CAD build for the part. Positions are in the model's coordinates, mm. A direction names the side the tool comes from. Give positions to 0.01 mm unless a question says otherwise; leave off trailing zeros. Order: outer loops, then holes, each group sorted by start corner. A loop starts at its lowest first (then second) coordinate and runs counter-clockwise, first axis right, second up. Notation, with made-up numbers: M 60,40.5 L 108,40.5 A27 cw 108,72.5 Z; hole C 73.5,-19.75 d2. An arc over 180 degrees is marked long. Put each result on its own line as item: value. Start each with the question number.
1) Cut at C-C (y = -19). Write the cut outline in (x, z), and give its area (3 significant figures).
2) Drill centre lines: line 1 (Z direction, x = 23, y = 12); line 2 (Y direction, x = 0, z = 4.5); line 3 (Y direction, x = -17.5, z = 1.25). Where is each one in solid material? Low to high. Write a range as [from, to].
3) Two-plate mould, pull along X, no slides. Class faces 1 (the face through (0, 0, 0)), 2 (the face through (-8.75, 28, 3)), 3 (the face through (0, 0, -2)): released by +X, released by -X, zero draft, split by the parting line, or undercut.
4) Cut at A-A (x = 0). Write the cut outline in (y, z), and give its area (3 significant figures).
5) Tool access for faces 4 (the face through (9, -27.5, 10)), 5 (the face through (8.75, 28, 3)): list every direction of +Z, -Z, +X, -X, +Y, -Y with a clear straight run to the whole face (end or side of a thin tool).
6) Cut at D-D (x = 20). Write the cut outline in (y, z), and give its area (3 significant figures).
7) Cut at B-B (z = 9.25). Write the cut outline in (x, y).
8) Pin check, flat tips, straight feed: pin 1 (1.6 mm diameter, centred on x = -3, z = -0.5, fed in from +Y); pin 2 (5 mm diameter, centred on x = 7.5, z = 5.5, fed in from -Y); pin 3 (1.5 mm diameter, centred on x = 17.5, z = 4.5, fed in from -Y). Stop position of each tip, or through.
```python
from build123d import *

# Parameters (mm, degrees)
F1_DEPTH      = 2
F2_DEPTH      = 10
F3_DEPTH      = 2.001
F4_DEPTH      = 25
F4_DEPTH_BACK = 25


with BuildPart() as f1:
    # F0 (on Top) → F1 (new body)
    with BuildSketch(Plane.XY):
        with BuildLine():
            Line((8.75, 27.3861278753), (8.75, 29.7394939432))
            ThreePointArc((8.75, 29.7394939432), (0, 31), (-8.75, 29.7394939432))
            Line((-8.75, 29.7394939432), (-8.75, 27.3861278753))
            ThreePointArc((-8.75, 27.3861278753), (0, 28.75), (8.75, 27.3861278753))
        make_face()
        with BuildLine():
            ThreePointArc((-8.75, 29.7394939432), (-18.5708104293, -24.821865361), (31, 0))
            ThreePointArc((31, 0), (24.821865361, 18.5708104293), (8.75, 29.7394939432))
            Line((8.75, 29.7394939432), (8.75, 27.3861278753))
            ThreePointArc((8.75, 27.3861278753), (23.2177195263, 16.9558249578), (28.75, 0))
            ThreePointArc((28.75, 0), (-16.9558249578, -23.2177195263), (-8.75, 27.3861278753))
            Line((-8.75, 27.3861278753), (-8.75, 29.7394939432))
        make_face()
        with BuildLine():
            Line((8.75, 22.0912080258), (8.75, 27.3861278753))
            ThreePointArc((8.75, 27.3861278753), (0, 28.75), (-8.75, 27.3861278753))
            Line((-8.75, 27.3861278753), (-8.75, 22.0912080258))
            Line((-8.75, 22.0912080258), (8.75, 22.0912080258))
        make_face()
        with BuildLine():
            ThreePointArc((28.75, 0), (23.2177195263, 16.9558249578), (8.75, 27.3861278753))
            Line((8.75, 27.3861278753), (8.75, 22.0912080258))
            Line((8.75, 22.0912080258), (-8.75, 22.0912080258))
            Line((-8.75, 22.0912080258), (-8.75, 27.3861278753))
            ThreePointArc((-8.75, 27.3861278753), (-16.9558249578, -23.2177195263), (28.75, 0))
        make_face()
    extrude(amount=-F1_DEPTH)

    # F0 (on Top) → F2 (join)
    with BuildSketch(Plane.XY):
        with BuildLine():
            Line((8.75, 27.3861278753), (8.75, 29.7394939432))
            ThreePointArc((8.75, 29.7394939432), (0, 31), (-8.75, 29.7394939432))
            Line((-8.75, 29.7394939432), (-8.75, 27.3861278753))
            ThreePointArc((-8.75, 27.3861278753), (0, 28.75), (8.75, 27.3861278753))
        make_face()
        with BuildLine():
            ThreePointArc((-8.75, 29.7394939432), (-18.5708104293, -24.821865361), (31, 0))
            ThreePointArc((31, 0), (24.821865361, 18.5708104293), (8.75, 29.7394939432))
            Line((8.75, 29.7394939432), (8.75, 27.3861278753))
            ThreePointArc((8.75, 27.3861278753), (23.2177195263, 16.9558249578), (28.75, 0))
            ThreePointArc((28.75, 0), (-16.9558249578, -23.2177195263), (-8.75, 27.3861278753))
            Line((-8.75, 27.3861278753), (-8.75, 29.7394939432))
        make_face()
    extrude(amount=F2_DEPTH)

    # F0 (on Top) → F3 (cut, through all)
    with BuildSketch(Plane.XY):
        with BuildLine():
            Line((8.75, 22.0912080258), (8.75, 27.3861278753))
            ThreePointArc((8.75, 27.3861278753), (0, 28.75), (-8.75, 27.3861278753))
            Line((-8.75, 27.3861278753), (-8.75, 22.0912080258))
            Line((-8.75, 22.0912080258), (8.75, 22.0912080258))
        make_face()
        with BuildLine():
            ThreePointArc((-8.75, 29.7394939432), (0, 31), (8.75, 29.7394939432))
            Line((8.75, 29.7394939432), (8.75, 35.3688262403))
            Line((8.75, 35.3688262403), (-8.75, 35.3688262403))
            Line((-8.75, 35.3688262403), (-8.75, 29.7394939432))
        make_face()
        with BuildLine():
            Line((8.75, 27.3861278753), (8.75, 29.7394939432))
            ThreePointArc((8.75, 29.7394939432), (0, 31), (-8.75, 29.7394939432))
            Line((-8.75, 29.7394939432), (-8.75, 27.3861278753))
            ThreePointArc((-8.75, 27.3861278753), (0, 28.75), (8.75, 27.3861278753))
        make_face()
    extrude(amount=-F3_DEPTH, mode=Mode.SUBTRACT)

    # F0 (on Top) → F4 (cut, two sides)
    with BuildSketch(Plane.XY) as f4_sk:
        with BuildLine():
            Line((8.75, 27.3861278753), (8.75, 29.7394939432))
            ThreePointArc((8.75, 29.7394939432), (0, 31), (-8.75, 29.7394939432))
            Line((-8.75, 29.7394939432), (-8.75, 27.3861278753))
            ThreePointArc((-8.75, 27.3861278753), (0, 28.75), (8.75, 27.3861278753))
        make_face()
    extrude(amount=-F4_DEPTH, mode=Mode.SUBTRACT)
    extrude(f4_sk.sketch, amount=F4_DEPTH_BACK, mode=Mode.SUBTRACT)


solid = f1.part
```
Solution:
1. outline: M -24.49,-2 L 24.49,-2 L 24.49,10 L 21.58,10 L 21.58,0 L -21.58,0 L -21.58,10 L -24.49,10 Z
1. area: 156 mm²
2. line 1: [-2, 0]
2. line 2: [-31, -28.75]
2. line 3: [-25.59, -22.81], [22.81, 25.59]
3. face 1: undercut
3. face 2: undercut
3. face 3: zero draft
4. outline: M -31,-2 L 22.09,-2 L 22.09,0 L -28.75,0 L -28.75,10 L -31,10 Z
4. area: 129 mm²
5. face 4: +Z, +X, -X, +Y, -Y
5. face 5: +Z, -Z, +Y
6. outline: M -23.69,-2 L 23.69,-2 L 23.69,10 L 20.65,10 L 20.65,0 L -20.65,0 L -20.65,10 L -23.69,10 Z
6. area: 155 mm²
7. outline: M -8.75,27.39 L -8.75,29.74 A31 ccw long 8.75,29.74 L 8.75,27.39 A28.75 cw long Z
8. pin 1: y = 22.09
8. pin 2: y = -30.59
8. pin 3: y = -26.09
